The listing builds one solid part. Answer for the finished solid, in the listing's coordinates (mm). Face numbers are marked on the shaded views. A direction names the side the tool comes from. Give positions to 0.01 mm unless a question says otherwise; leave off trailing zeros. Order: outer loops, then holes, each group sorted by start corner. A loop starts at its lowest first (then second) coordinate and runs counter-clockwise, first axis right, second up. Notation, with made-up numbers: (16.25, 25) - (23.25, 25) arc R8 ccw to (23.25, 34) - close; hole circle Ø11 at (43.5, 58.25). An arc over 180 degrees is marked (long way). Answer as CSV lines item,"result". Start each with the question number.
1. Which of the six approach directions +Z, -Z, +X, -X, +Y, -Y give full straight-line access (tool end or side, diameter ignored) to the marked faces 4 and 5?
2. Section A-A on z = 0 is taken. Give the vertices of the cut face in (x, y).
3. Consider line 1 along X through (y, z) = (0.25, 0); line 2 along Z through (x, y) = (8, 0.25); line 3 along Y through (x, z) = (2.5, -0.5). Determine where each line is inside the solid, lowest interval first. Write a range as [from, to].
4. Flat-ended cylindrical pins translate along their axes: pin 1 (3 mm diameter, centred on x = 8, z = 2, fed in from -Y); pin 2 (1.5 mm diameter, centred on x = 10.5, z = 1.5, fed in from +Y); pin 3 (1.7 mm diameter, centred on x = 8, z = 0, fed in from +Y). Find the tip coordinate at first contact, or state that the pin passes through.
5. Section C-C on z = 1.75 is taken. Give the vertices of the cut face in (x, y).
6. Section D-D on y = 2 is taken. Give the vertices of the cut face in (x, z).
7. Section B-B on x = 2.5 is taken. Give the vertices of the cut face in (y, z), and give its area (4 significant figures).
8. Determine the mould class of the marked faces 1, 2 and 3 for opening direction X: +X half, -X half, draft (parallel to the pull), parting line (faces both ways), or undercut.
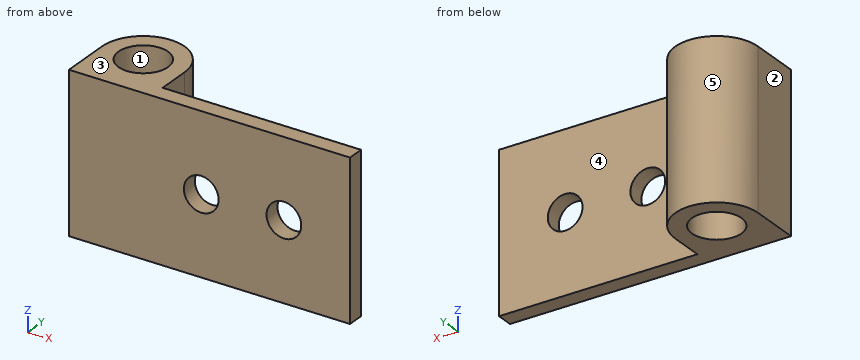
Autodesk Inventor part; units mm, degrees
ref_plane "A_XY" through (2.5, 3, 0) normal (0, 0, 1) x (1, 0, 0)
ref_plane "A_YZ" through (2.5, 3, 0) normal (1, 0, 0) x (0, 1, 0)
ref_plane "A_ZX" through (2.5, 3, 0) normal (0, 1, 0) x (0, 0, 1)
sketch "Sketch_1" plane through (0, 0, 0) normal (0, 0, 1) x (1, 0, 0)
  line L0 (0, 3) -> (0, 0)
  line L1 (0, 0) -> (17, 0)
  line L2 (17, 0) -> (17, 1)
  line L3 (17, 1) -> (5, 1)
  line L4 (5, 1) -> (5, 3)
  arc A0 (5, 3) -> (0, 3) centre (2.5, 3) ccw
  circle A1 centre (2.5, 3) radius 1.5
extrude "Extrusion1" add sketch "Sketch_1" along normal mid plane 9.5
sketch "Sketch_2" plane through (0, 0, 0) normal (0, 1, 0) x (-1, 0, 0)
  circle A0 centre (-8, 0) radius 1.05
extrude "Extrusion2" cut sketch "Sketch_2" along normal mid plane 9.5
sketch "Sketch_3" plane through (0, 0, 0) normal (0, 1, 0) x (-1, 0, 0)
  circle A0 centre (-13, 0) radius 1.05
extrude "Extrusion3" cut sketch "Sketch_3" along normal mid plane 9.5
ref_plane "A_XY" through (2.5, 3, 0) normal (0, 0, 1) x (1, 0, 0)
ref_plane "A_YZ" through (2.5, 3, 0) normal (1, 0, 0) x (0, 1, 0)
ref_plane "A_ZX" through (2.5, 3, 0) normal (0, 1, 0) x (0, 0, 1)
properties part number "PKWS1_b"
Checks:
1,face 4,"+Z, -Z, +X, +Y"
1,face 5,"+Z, -Z, +Y"
2,outline,"(0, 0) - (6.95, 0) - (6.95, 1) - (5, 1) - (5, 3) arc R2.5 ccw to (0, 3) - close; (9.05, 0) - (11.95, 0) - (11.95, 1) - (9.05, 1) - close; (14.05, 0) - (17, 0) - (17, 1) - (14.05, 1) - close; hole circle Ø3 at (2.5, 3)"
3,line 1,"x = [0, 6.95], [9.05, 11.95], [14.05, 17]"
3,line 2,"z = [-4.75, -1.05], [1.05, 4.75]"
3,line 3,"y = [0, 1.5], [4.5, 5.5]"
4,pin 1,"stops at y = 0"
4,pin 2,"stops at y = 1"
4,pin 3,"passes through"
5,outline,"(0, 0) - (17, 0) - (17, 1) - (5, 1) - (5, 3) arc R2.5 ccw to (0, 3) - close; hole circle Ø3 at (2.5, 3)"
6,outline,"(0, -4.75) - (1.38, -4.75) - (1.38, 4.75) - (0, 4.75) - close; (3.62, -4.75) - (5, -4.75) - (5, 4.75) - (3.62, 4.75) - close"
7,outline,"(0, -4.75) - (1.5, -4.75) - (1.5, 4.75) - (0, 4.75) - close; (4.5, -4.75) - (5.5, -4.75) - (5.5, 4.75) - (4.5, 4.75) - close"
7,area,"23.75 mm²"
8,face 1,"undercut"
8,face 2,"-X half"
8,face 3,"draft"
